```python
from build123d import *

# Parameters (mm, degrees)
F1_DEPTH    = 3.175
F2_W        = 3.175
F2_H        = 3.175
F3_DEPTH    = 25.4
F4_T1_DEPTH = 19.0841031127


# Not quite as in the source:
# - a fillet or chamfer that OpenCascade refuses, or shapes differently, is made with other operations: its cross-section is extruded or revolved along the edge and cut away or added


with BuildPart() as f1:
    # F0 (on Right) → F1 (new body)
    with BuildSketch(Plane.YZ):
        with BuildLine():
            ThreePointArc((17.7183197491, -6.9974027515), (11.9270078227, 0), (17.7183197491, 6.9974027515))
            ThreePointArc((17.7183197491, 6.9974027515), (16.4977839421, 9.525), (14.9190884179, 11.8458136394))
            ThreePointArc((14.9190884179, 11.8458136394), (5.9635039114, 10.3290917656), (2.7992313312, 18.8432163909))
            ThreePointArc((2.7992313312, 18.8432163909), (0, 19.05), (-2.7992313312, 18.8432163909))
            ThreePointArc((-2.7992313312, 18.8432163909), (-2.5020157635, 17.6871997533), (-2.4020078227, 16.4977839421))
            ThreePointArc((-2.4020078227, 16.4977839421), (-7.0435721899, 9.8209932773), (-14.9190884179, 11.8458136394))
            ThreePointArc((-14.9190884179, 11.8458136394), (-16.4977839421, 9.525), (-17.7183197491, 6.9974027515))
            ThreePointArc((-17.7183197491, 6.9974027515), (-13.5626251464, 4.5415564264), (-11.9270078227, 0))
            ThreePointArc((-11.9270078227, 0), (-13.5626251464, -4.5415564264), (-17.7183197491, -6.9974027515))
            ThreePointArc((-17.7183197491, -6.9974027515), (-16.4977839421, -9.525), (-14.9190884179, -11.8458136394))
            ThreePointArc((-14.9190884179, -11.8458136394), (-7.0435721899, -9.8209932773), (-2.4020078227, -16.4977839421))
            ThreePointArc((-2.4020078227, -16.4977839421), (-2.5020157635, -17.6871997533), (-2.7992313312, -18.8432163909))
            ThreePointArc((-2.7992313312, -18.8432163909), (0, -19.05), (2.7992313312, -18.8432163909))
            ThreePointArc((2.7992313312, -18.8432163909), (5.9635039114, -10.3290917656), (14.9190884179, -11.8458136394))
            ThreePointArc((14.9190884179, -11.8458136394), (16.4977839421, -9.525), (17.7183197491, -6.9974027515))
        make_face()
    extrude(amount=F1_DEPTH)

    # F2 (on face) → F3 (cut)
    with BuildSketch(Plane(origin=(0, 0, 0), x_dir=(0, -1, 0), z_dir=(-1, 0, 0))):
        Rectangle(F2_W, F2_H)
    extrude(amount=-F3_DEPTH, mode=Mode.SUBTRACT)

    # F4: fillet of radius 2.7258813335 on 12 edges, made by hand

    # F4_s2 → F4_t1 (cut)
    with BuildSketch(Plane.YZ.offset(-7.9545515563)):
        with BuildLine():
            ThreePointArc((-16.6826195947, 9.1974291766), (-15.0505041811, 10.5005937812), (-12.9751564545, 10.2661358457))
            ThreePointArc((-12.9751564545, 10.2661358457), (-14.0171055557, 10.9698543809), (-14.9190884179, 11.8458136394))
            ThreePointArc((-14.9190884179, 11.8458136394), (-15.8562439561, 10.5585049892), (-16.6826195947, 9.1974291766))
        make_face()
        with BuildLine():
            ThreePointArc((-15.3783126684, 6.1037471848), (-16.6190330599, 7.78382207), (-16.3065171138, 9.8488577824))
            ThreePointArc((-16.3065171138, 9.8488577824), (-17.0720555246, 8.45265758), (-17.7183197491, 6.9974027515))
            ThreePointArc((-17.7183197491, 6.9974027515), (-16.5087253475, 6.6542423084), (-15.3783126684, 6.1037471848))
        make_face()
        with BuildLine():
            ThreePointArc((-16.3065171138, -9.8488577824), (-16.6190330599, -7.78382207), (-15.3783126684, -6.1037471848))
            ThreePointArc((-15.3783126684, -6.1037471848), (-16.5087253475, -6.6542423084), (-17.7183197491, -6.9974027515))
            ThreePointArc((-17.7183197491, -6.9974027515), (-17.0720555246, -8.45265758), (-16.3065171138, -9.8488577824))
        make_face()
        with BuildLine():
            ThreePointArc((-12.9751564545, -10.2661358457), (-15.0505041811, -10.5005937812), (-16.6826195947, -9.1974291766))
            ThreePointArc((-16.6826195947, -9.1974291766), (-15.8562439561, -10.5585049892), (-14.9190884179, -11.8458136394))
            ThreePointArc((-14.9190884179, -11.8458136394), (-14.0171055557, -10.9698543809), (-12.9751564545, -10.2661358457))
        make_face()
        with BuildLine():
            ThreePointArc((-2.4031562138, -16.3698830306), (-1.5685288788, -18.2844158512), (0.3761024809, -19.046286959))
            ThreePointArc((0.3761024809, -19.046286959), (-1.2158115686, -19.0111625691), (-2.7992313312, -18.8432163909))
            ThreePointArc((-2.7992313312, -18.8432163909), (-2.4916197918, -17.6240966892), (-2.4031562138, -16.3698830306))
        make_face()
        with BuildLine():
            ThreePointArc((-2.4031562138, 16.3698830306), (-1.5685288788, 18.2844158512), (0.3761024809, 19.046286959))
            ThreePointArc((0.3761024809, 19.046286959), (-1.2158115686, 19.0111625691), (-2.7992313312, 18.8432163909))
            ThreePointArc((-2.7992313312, 18.8432163909), (-2.4916197918, 17.6240966892), (-2.4031562138, 16.3698830306))
        make_face()
        with BuildLine():
            ThreePointArc((16.6826195947, 9.1974291766), (15.0505041811, 10.5005937812), (12.9751564545, 10.2661358457))
            ThreePointArc((12.9751564545, 10.2661358457), (14.0171055557, 10.9698543809), (14.9190884179, 11.8458136394))
            ThreePointArc((14.9190884179, 11.8458136394), (15.8562439561, 10.5585049892), (16.6826195947, 9.1974291766))
        make_face()
        with BuildLine():
            ThreePointArc((-0.3761024809, 19.046286959), (1.5685288788, 18.2844158512), (2.4031562138, 16.3698830306))
            ThreePointArc((2.4031562138, 16.3698830306), (2.4916197918, 17.6240966892), (2.7992313312, 18.8432163909))
            ThreePointArc((2.7992313312, 18.8432163909), (1.2158115686, 19.0111625691), (-0.3761024809, 19.046286959))
        make_face()
        with BuildLine():
            ThreePointArc((15.3783126684, 6.1037471848), (16.6190330599, 7.78382207), (16.3065171138, 9.8488577824))
            ThreePointArc((16.3065171138, 9.8488577824), (17.0720555246, 8.45265758), (17.7183197491, 6.9974027515))
            ThreePointArc((17.7183197491, 6.9974027515), (16.5087253475, 6.6542423084), (15.3783126684, 6.1037471848))
        make_face()
        with BuildLine():
            ThreePointArc((16.3065171138, -9.8488577824), (16.6190330599, -7.78382207), (15.3783126684, -6.1037471848))
            ThreePointArc((15.3783126684, -6.1037471848), (16.5087253475, -6.6542423084), (17.7183197491, -6.9974027515))
            ThreePointArc((17.7183197491, -6.9974027515), (17.0720555246, -8.45265758), (16.3065171138, -9.8488577824))
        make_face()
        with BuildLine():
            ThreePointArc((12.9751564545, -10.2661358457), (15.0505041811, -10.5005937812), (16.6826195947, -9.1974291766))
            ThreePointArc((16.6826195947, -9.1974291766), (15.8562439561, -10.5585049892), (14.9190884179, -11.8458136394))
            ThreePointArc((14.9190884179, -11.8458136394), (14.0171055557, -10.9698543809), (12.9751564545, -10.2661358457))
        make_face()
        with BuildLine():
            ThreePointArc((-0.3761024809, -19.046286959), (1.5685288788, -18.2844158512), (2.4031562138, -16.3698830306))
            ThreePointArc((2.4031562138, -16.3698830306), (2.4916197918, -17.6240966892), (2.7992313312, -18.8432163909))
            ThreePointArc((2.7992313312, -18.8432163909), (1.2158115686, -19.0111625691), (-0.3761024809, -19.046286959))
        make_face()
    extrude(amount=F4_T1_DEPTH, mode=Mode.SUBTRACT)


solid = f1.part
```
The listing builds one solid part. Answer for the finished solid, in the listing's coordinates (mm). A direction names the side the tool comes from. Round coordinates to 2 decimals unless told otherwise and drop trailing zeros. Loops run counter-clockwise (first coordinate to the right, second up) from the corner with the lowest first, then second, coordinate; pieces in that order, holes last.
1) A cutting plane is placed at C-C on z = 15. Determine the outline of the cut face in (x, y) (3 decimals), plus the area to 3 significant figures.
Outcome:
outline: (0, -2.561) - (3.175, -2.561) - (3.175, 2.561) - (0, 2.561) - close
area: 16.3 mm2
2) For a pull along Z with two mould halves and no side action, classify faces 3 (the face through (1.565, -14.841, -10.552)), 4 (the face through (1.57, 16.56, 7.58)), 5 (the face through (1.565, -1.718, 18.129)) as released by +Z, released by -Z, zero draft, split by the parting line, or undercut.
Outcome:
face 3: released by -Z
face 4: undercut
face 5: released by +Z
3) A cutting plane is placed at A-A on z = -1. Determine the outline of the cut face in (x, y) (1 decimal), plus the area to 3 significant figures.
Outcome:
outline: (0, -12) - (3.2, -12) - (3.2, -1.6) - (0, -1.6) - close; (0, 1.6) - (3.2, 1.6) - (3.2, 12) - (0, 12) - close
area: 66.1 mm2
4) For faces 1 (the face through (2, -1.588, 0)), 2 (the face through (1.565, -16.576, -7.629)), determine the directions among +Z, -Z, +X, -X, +Y, -Y from which every point of the face is accessible in a straight line to the end or side of a thin tool.
Outcome:
face 1: +X, -X
face 2: +X, -X, -Y
5) A cutting plane is placed at D-D on y = -10. Determine the outline of the cut face in (x, z) (3 decimals).
Outcome:
outline: (0, -9.391) - (3.175, -9.391) - (3.175, 9.391) - (0, 9.391) - close
6) Consider line 1 (Z direction, x = 2.1, y = 12.5); line 2 (Y direction, x = 2.3, z = 1); line 3 (Z direction, x = 3.05, y = 13.5). Determine where each line is inside the solid, lowest interval first.
Outcome:
line 1: z = -10.03 to -2.8, 2.8 to 10.03
line 2: y = -12 to -1.59, 1.59 to 12
line 3: z = -10.49 to -4.46, 4.46 to 10.49
7) Given P1, Ø1, axis at x = 1, z = -0.5, coming from the +Y side; P2, Ø1.5, axis at x = 1.5, y = -5.5, coming from the -Z side, each flat-ended and moving along its own axis, determine where each tip first touches the part or whether it passes through.
Outcome:
P1: stops at y = 12
P2: stops at z = -11.21
